Build history of the part. All positions in model axes, mm. Face numbers are marked on the shaded views. A direction names the side the tool comes from. Give positions to 0.01 mm unless a question says otherwise; leave off trailing zeros. Write each loop counter-clockwise with the first axis right and the second up, starting at its lowest first coordinate (ties: lowest second). Pieces come first, ordered by that corner, then holes. Notation, with made-up numbers: (44.5, 72) -> (70.5, 72) arc R12 cw to (70.5, 84) -> close; hole circle Ø9 at (75, 21). An arc over 180 degrees is marked (long way). One line per question, with ' | ' between items. Start each with the question number.
(1) Band-saw the part on C-C, the plane x = 18. Give the cut face in (y, z).
(2) Band-saw the part on A-A, the plane x = 25.5. Give the cut face in (y, z), and give its area (3 significant figures).
(3) Tool access for the marked faces 1, 2, 3, 4 and 5: list every direction of +Z, -Z, +X, -X, +Y, -Y with a clear straight run to the whole face (end or side of a thin tool).
(4) Band-saw the part on D-D, the plane z = -57.5. Give the cut face in (x, y), and give its area (3 significant figures).
(5) Drill centre lines: probe 1 along Z at (x, y) = (3, 6); probe 2 along X at (y, z) = (3, 3); probe 3 along X at (y, z) = (-2, -25). Where is each one in solid material? Low to high. Write a range as from..to.
(6) Pin check, flat tips, straight feed: P1, Ø2, axis at x = 22, z = -31.5, coming from the -Y side; P2, Ø10, axis at x = 27, z = -6.5, coming from the -Y side; P3, Ø5, axis at x = 30, z = -35.5, coming from the +Y side; P4, Ø3, axis at x = 31.5, z = -51, coming from the -Y side. Stop position of each tip, or through.
(7) Band-saw the part on B-B, the plane y = 9. Give the cut face in (x, z).
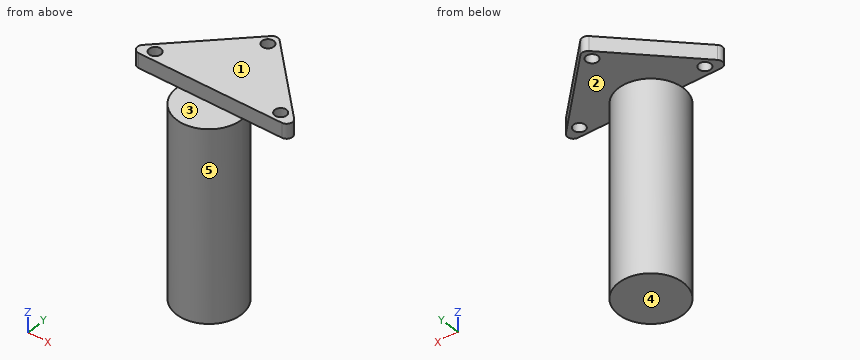
from build123d import *

# Parameters (mm, degrees)
SKETCH_R     = 2
PAD_DEPTH    = 5
SKETCH001_R  = 11
PAD001_DEPTH = 65


with BuildPart() as part:
    # Sketch → Pad (new body)
    with BuildSketch(Plane.XY):
        with BuildLine():
            Line((1.414214, 0), (49.84062, 0))
            ThreePointArc((49.84062, 0), (51.688379, 1.234633), (51.254834, 3.414214))
            Line((51.254834, 3.414214), (27.041631, 27.627417))
            ThreePointArc((27.041631, 27.627417), (25.627417, 28.213203), (24.213203, 27.627417))
            Line((0, 3.414214), (24.213203, 27.627417))
            ThreePointArc((0, 3.414214), (-0.433546, 1.234633), (1.414214, 0))
        make_face()
        with Locations((4.414214, 3.25)):
            Circle(SKETCH_R, mode=Mode.SUBTRACT)
        with Locations((46.84062, 3.25)):
            Circle(SKETCH_R, mode=Mode.SUBTRACT)
        with Locations((25.627417, 24.463203)):
            Circle(SKETCH_R, mode=Mode.SUBTRACT)
    extrude(amount=PAD_DEPTH)

    # Sketch001 (on Face10 of Pad) → Pad001 (join)
    with BuildSketch(Plane(origin=(0, 0, 0), x_dir=(1, 0, 0), z_dir=(0, 0, -1))):
        with Locations((25.627417, 0.536797)):
            Circle(SKETCH001_R)
    extrude(amount=PAD001_DEPTH)


solid = part.part
Results:
1) outline: (-8.46, -65) -> (7.39, -65) -> (7.39, 0) -> (21.41, 0) -> (21.41, 5) -> (0, 5) -> (0, 0) -> (-8.46, 0) -> close
2) outline: (-11.54, -65) -> (10.46, -65) -> (10.46, 0) -> (22.47, 0) -> (22.47, 5) -> (0, 5) -> (0, 0) -> (-11.54, 0) -> close; (26.46, 0) -> (28.21, 0) -> (28.21, 5) -> (26.46, 5) -> close | area: 1,550 mm²
3) face 1: +Z, +X, -X, +Y, -Y | face 2: -Z, +Y | face 3: +Z, +X, -X, -Y | face 4: -Z, +X, -X, +Y, -Y | face 5: -Z
4) outline: circle Ø22 at (25.63, -0.54) | area: 380 mm²
5) probe 1: z = 0..5 | probe 2: x = -0.32..2.43, 6.4..44.86, 48.82..51.57 | probe 3: x = 14.73..36.53
6) P1: stops at y = -11.22 | P2: stops at y = -11.54 | P3: stops at y = 10.3 | P4: stops at y = -10.63
7) outline: (5.59, 0) -> (20.15, 0) -> (20.15, -65) -> (31.11, -65) -> (31.11, 0) -> (45.67, 0) -> (45.67, 5) -> (5.59, 5) -> close
